from build123d import *

# Parameters (mm, degrees)
SKETCH1_R           = 2.6035
BOSS_EXTRUDE1_DEPTH = 104.775


with BuildPart() as part:
    # Sketch1 → Boss-Extrude1 (new body)
    with BuildSketch(Plane(origin=(0, 0, 0), x_dir=(0, 0, -1), z_dir=(0, 1, 0))):
        with BuildLine():
            Line((6.333126718, -12.7), (9.550443118, -12.7))
            ThreePointArc((9.550443118, -12.7), (10.058366869, -12.192000006), (10.566443095, -12.699847501))
            ThreePointArc((10.566443095, -12.699847501), (12.082537762, -12.08250727), (12.699846982, -10.566399977))
            ThreePointArc((12.699846982, -10.566399977), (12.192000006, -10.058323491), (12.7, -9.5504))
            Line((12.7, -9.5504), (12.7, -6.3330836))
            ThreePointArc((12.7, -6.3330836), (12.192, -5.8250836), (12.7, -5.3170836))
            Line((12.7, -5.3170836), (12.7, -4.287469289))
            ThreePointArc((12.7, -4.287469289), (12.39275138, -3.545705502), (11.650987593, -3.238456882))
            Line((11.650987593, -3.238456882), (11.539212407, -3.238456882))
            ThreePointArc((11.539212407, -3.238456882), (10.79744862, -3.545705502), (10.4902, -4.287469289))
            Line((10.4902, -4.287469289), (10.4902, -6.402089023))
            ThreePointArc((10.4902, -6.402089023), (9.856505071, -7.351067942), (8.737131347, -7.129408934))
            Line((8.737131347, -7.129408934), (5.441005833, -3.840816462))
            ThreePointArc((5.441005833, -3.840816462), (4.750877967, -2.809883091), (4.5085, -1.593185507))
            Line((4.5085, -1.593185507), (4.5085, 1.593185507))
            ThreePointArc((4.5085, 1.593185507), (4.750877967, 2.809883091), (5.441005833, 3.840816462))
            Line((5.441005833, 3.840816462), (8.737131347, 7.129408934))
            ThreePointArc((8.737131347, 7.129408934), (9.856505071, 7.351067942), (10.4902, 6.402089023))
            Line((10.4902, 6.402089023), (10.4902, 4.287469289))
            ThreePointArc((10.4902, 4.287469289), (10.79744862, 3.545705502), (11.539212407, 3.238456882))
            Line((11.539212407, 3.238456882), (11.650987593, 3.238456882))
            ThreePointArc((11.650987593, 3.238456882), (12.39275138, 3.545705502), (12.7, 4.287469289))
            Line((12.7, 4.287469289), (12.7, 5.3170836))
            ThreePointArc((12.7, 5.3170836), (12.192, 5.8250836), (12.7, 6.3330836))
            Line((12.7, 6.3330836), (12.7, 9.5504))
            ThreePointArc((12.7, 9.5504), (12.192000006, 10.058323491), (12.699846982, 10.566399977))
            ThreePointArc((12.699846982, 10.566399977), (12.082537762, 12.08250727), (10.566443095, 12.699847501))
            ThreePointArc((10.566443095, 12.699847501), (10.058366869, 12.192000006), (9.550443118, 12.7))
            Line((9.550443118, 12.7), (6.333126718, 12.7))
            ThreePointArc((6.333126718, 12.7), (5.825126718, 12.192), (5.317126718, 12.7))
            Line((5.317126718, 12.7), (4.287512407, 12.7))
            ThreePointArc((4.287512407, 12.7), (3.54574862, 12.39275138), (3.2385, 11.650987593))
            Line((3.2385, 11.650987593), (3.2385, 11.539212407))
            ThreePointArc((3.2385, 11.539212407), (3.54574862, 10.79744862), (4.287512407, 10.4902))
            Line((4.287512407, 10.4902), (6.476788598, 10.4902))
            ThreePointArc((6.476788598, 10.4902), (7.432222385, 9.85140422), (7.207036008, 8.724370562))
            Line((7.207036008, 8.724370562), (3.898272566, 5.423169045))
            ThreePointArc((3.898272566, 5.423169045), (2.869120213, 4.736787962), (1.655778399, 4.4958))
            Line((1.655778399, 4.4958), (-1.655778399, 4.4958))
            ThreePointArc((-1.655778399, 4.4958), (-2.869120213, 4.736787962), (-3.898272566, 5.423169045))
            Line((-3.898272566, 5.423169045), (-7.207036008, 8.724370562))
            ThreePointArc((-7.207036008, 8.724370562), (-7.432222385, 9.85140422), (-6.476788598, 10.4902))
            Line((-6.476788598, 10.4902), (-4.287512407, 10.4902))
            ThreePointArc((-4.287512407, 10.4902), (-3.54574862, 10.79744862), (-3.2385, 11.539212407))
            Line((-3.2385, 11.539212407), (-3.2385, 11.650987593))
            ThreePointArc((-3.2385, 11.650987593), (-3.54574862, 12.39275138), (-4.287512407, 12.7))
            Line((-4.287512407, 12.7), (-5.317126718, 12.7))
            ThreePointArc((-5.317126718, 12.7), (-5.825126718, 12.192), (-6.333126718, 12.7))
            Line((-6.333126718, 12.7), (-9.550443118, 12.7))
            ThreePointArc((-9.550443118, 12.7), (-10.058366869, 12.192000006), (-10.566443095, 12.699847501))
            ThreePointArc((-10.566443095, 12.699847501), (-12.082537762, 12.08250727), (-12.699846982, 10.566399977))
            ThreePointArc((-12.699846982, 10.566399977), (-12.192000006, 10.058323491), (-12.7, 9.5504))
            Line((-12.7, 9.5504), (-12.7, 6.3330836))
            ThreePointArc((-12.7, 6.3330836), (-12.192, 5.8250836), (-12.7, 5.3170836))
            Line((-12.7, 5.3170836), (-12.7, 4.287469289))
            ThreePointArc((-12.7, 4.287469289), (-12.39275138, 3.545705502), (-11.650987593, 3.238456882))
            Line((-11.650987593, 3.238456882), (-11.539212407, 3.238456882))
            ThreePointArc((-11.539212407, 3.238456882), (-10.79744862, 3.545705502), (-10.4902, 4.287469289))
            Line((-10.4902, 4.287469289), (-10.4902, 6.402089023))
            ThreePointArc((-10.4902, 6.402089023), (-9.856505071, 7.351067942), (-8.737131347, 7.129408934))
            Line((-8.737131347, 7.129408934), (-5.441005833, 3.840816462))
            ThreePointArc((-5.441005833, 3.840816462), (-4.750877967, 2.809883091), (-4.5085, 1.593185507))
            Line((-4.5085, 1.593185507), (-4.5085, -1.593185507))
            ThreePointArc((-4.5085, -1.593185507), (-4.750877967, -2.809883091), (-5.441005833, -3.840816462))
            Line((-5.441005833, -3.840816462), (-8.737131347, -7.129408934))
            ThreePointArc((-8.737131347, -7.129408934), (-9.856505071, -7.351067942), (-10.4902, -6.402089023))
            Line((-10.4902, -6.402089023), (-10.4902, -4.287469289))
            ThreePointArc((-10.4902, -4.287469289), (-10.79744862, -3.545705502), (-11.539212407, -3.238456882))
            Line((-11.539212407, -3.238456882), (-11.650987593, -3.238456882))
            ThreePointArc((-11.650987593, -3.238456882), (-12.39275138, -3.545705502), (-12.7, -4.287469289))
            Line((-12.7, -4.287469289), (-12.7, -5.3170836))
            ThreePointArc((-12.7, -5.3170836), (-12.192, -5.8250836), (-12.7, -6.3330836))
            Line((-12.7, -6.3330836), (-12.7, -9.5504))
            ThreePointArc((-12.7, -9.5504), (-12.192000006, -10.058323491), (-12.699846982, -10.566399977))
            ThreePointArc((-12.699846982, -10.566399977), (-12.082537762, -12.08250727), (-10.566443095, -12.699847501))
            ThreePointArc((-10.566443095, -12.699847501), (-10.058366869, -12.192000006), (-9.550443118, -12.7))
            Line((-9.550443118, -12.7), (-6.333126718, -12.7))
            ThreePointArc((-6.333126718, -12.7), (-5.825126718, -12.192), (-5.317126718, -12.7))
            Line((-5.317126718, -12.7), (-4.287512407, -12.7))
            ThreePointArc((-4.287512407, -12.7), (-3.54574862, -12.39275138), (-3.2385, -11.650987593))
            Line((-3.2385, -11.650987593), (-3.2385, -11.539212407))
            ThreePointArc((-3.2385, -11.539212407), (-3.54574862, -10.79744862), (-4.287512407, -10.4902))
            Line((-4.287512407, -10.4902), (-6.416408329, -10.4902))
            ThreePointArc((-6.416408329, -10.4902), (-7.41473083, -9.822813117), (-7.179650497, -8.645192506))
            Line((-7.179650497, -8.645192506), (-3.952270251, -5.423690499))
            ThreePointArc((-3.952270251, -5.423690499), (-2.922936451, -4.736929036), (-1.709253557, -4.4958))
            Line((-1.709253557, -4.4958), (1.709253557, -4.4958))
            ThreePointArc((1.709253557, -4.4958), (2.922936451, -4.736929036), (3.952270251, -5.423690499))
            Line((3.952270251, -5.423690499), (7.179650497, -8.645192506))
            ThreePointArc((7.179650497, -8.645192506), (7.41473083, -9.822813117), (6.416408329, -10.4902))
            Line((6.416408329, -10.4902), (4.287512407, -10.4902))
            ThreePointArc((4.287512407, -10.4902), (3.54574862, -10.79744862), (3.2385, -11.539212407))
            Line((3.2385, -11.539212407), (3.2385, -11.650987593))
            ThreePointArc((3.2385, -11.650987593), (3.54574862, -12.39275138), (4.287512407, -12.7))
            Line((4.287512407, -12.7), (5.317126718, -12.7))
            ThreePointArc((5.317126718, -12.7), (5.825126718, -12.192), (6.333126718, -12.7))
        make_face()
        Circle(SKETCH1_R, mode=Mode.SUBTRACT)
    extrude(amount=BOSS_EXTRUDE1_DEPTH)


solid = part.part
For this review, take the finished solid that the model builds, in its own axes (mm). A direction names the side the tool comes from. Round coordinates to 2 decimals unless told otherwise and drop trailing zeros. Loops run counter-clockwise (first coordinate to the right, second up) from the corner with the lowest first, then second, coordinate; pieces in that order, holes last. Notation, with made-up numbers: (77.25, -16) - (134.25, -16) arc R17 cw to (134.25, 8) - close; hole circle Ø3 at (-32.75, -22.75). An arc over 180 degrees is marked (long way). One line per question, with ' | ' between items.
Q1. The part is to be moulded in two halves that separate along Z. For faces 4 (the flat face through (10.49, 52, 5)), 5 (the flat face through (-12.7, 52, 8)), 6 (the flat face through (8, 52, 12.7)), 7 (the flat face through (8, 52, -12.7)), say which applies: released by +Z, released by -Z, zero draft, split by the parting line, or undercut.
Taken from the geometry:
face 4: undercut | face 5: zero draft | face 6: released by +Z | face 7: released by -Z
Q2. Take a section at A-A (z = 0). Give the boundary of the cut face in (x, y) (1 decimal), and give its area (3 significant figures).
Taken from the geometry:
outline: (-4.5, 0) - (-2.6, 0) - (-2.6, 104.8) - (-4.5, 104.8) - close; (2.6, 0) - (4.5, 0) - (4.5, 104.8) - (2.6, 104.8) - close | area: 397 mm²
Q3. For pin 1 (1.7 mm diameter, centred on y = 40, z = 5.5, fed in from -X); pin 2 (4 mm diameter, centred on y = 78, z = 1, fed in from +X); pin 3 (3.5 mm diameter, centred on y = 53, z = 0, fed in from -X); pin 4 (1.6 mm diameter, centred on x = 0, y = 69.5, fed in from -Z), all flat-tipped, find the tip position at first contact; note any pin that passes through.
Taken from the geometry:
pin 1: stops at x = -12.7 | pin 2: stops at x = 4.77 | pin 3: stops at x = -4.5 | pin 4: stops at z = -4.51
Q4. For line 1 along Z through (x, y) = (0, 45.5); line 2 along X through (y, z) = (79.5, -5.25); line 3 along X through (y, z) = (50, 0), list the stretches that pass through material, from the lowest coordinate up. Write a range as [from, to].
Taken from the geometry:
line 1: z = [-4.51, -2.6], [2.6, 4.51] | line 2: x = [-12.7, -10.49], [-6.77, -3.63], [3.63, 6.72], [10.49, 12.7] | line 3: x = [-4.5, -2.6], [2.6, 4.5]
Q5. Take a section at B-B (x = 0). Give the boundary of the cut face in (y, z) (1 decimal), and give its area (3 significant figures).
Taken from the geometry:
outline: (0, -4.5) - (104.8, -4.5) - (104.8, -2.6) - (0, -2.6) - close; (0, 2.6) - (104.8, 2.6) - (104.8, 4.5) - (0, 4.5) - close | area: 399 mm²
Q6. Tool access review of faces 1 (the flat face through (-5, 52, -10.49)), 2 (the flat face through (-8, 52, -12.7)), 3 (the flat face through (0, 52, -4.508)): name each direction out of +Z, -Z, +X, -X, +Y, -Y from which nothing blocks a thin tool from reaching the whole face with its end or side.
Taken from the geometry:
face 1: +Y, -Y | face 2: -Z, +X, -X, +Y, -Y | face 3: -Z, +Y, -Y
